Geometry: see drawing. Coordinates: mm, zero at the bounding-box minimum. Give positions to 0.01 mm unless a question says otherwise; leave off trailing zeros. Order: outer loops, then holes, each group sorted by start corner. A loop starts at its lowest first (then second) coordinate and runs counter-clockwise, first axis right, second up. Notation, with made-up numbers: M 19,0 L 67,0 A30 ccw 67,39 Z; hole C 88,65.5 d11. An arc over 180 degrees is marked long. Use a Markdown table: item, result.
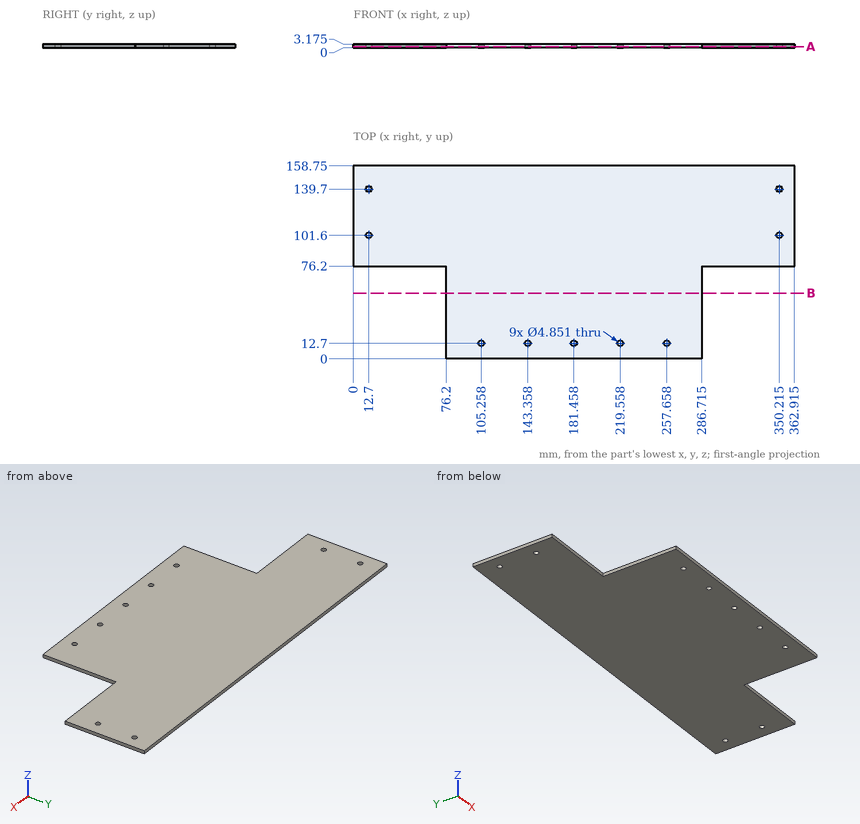
1) Cut plane B-B on y = 54. Return loops of the section in (x, z) (1 decimal).
Response values:
| item | result |
|---|---|
| outline | M 76.2,0 L 286.7,0 L 286.7,3.2 L 76.2,3.2 Z |
2) Material intervals for line 1 (X direction, y = 12.7, z = 1.5) (1 decimal); line 2 (X direction, y = 139.7, z = 2.05) (1 decimal); line 3 (X direction, y = 140.5, z = 0.5) (1 decimal), sorted ascending. Write a range as from..to.
Response values:
| item | result |
|---|---|
| line 1 | x = 76.2..102.8, 107.7..140.9, 145.8..179, 183.9..217.1, 222..255.2, 260.1..286.7 |
| line 2 | x = 0..10.3, 15.1..347.8, 352.6..362.9 |
| line 3 | x = 0..10.4, 15..347.9, 352.5..362.9 |
3) Cut plane A-A on z = 1.05. State how many separate pieces and enclosed holes the cut face has, and give its area (3 significant figures).
Response values:
| item | result |
|---|---|
| separate pieces | 1 |
| enclosed holes | 9 |
| area | 45,800 mm² |
4) First-contact query: pin 1 Ø3 at (x, y) = (350.22, 101.6) entering from -Z; pin 2 Ø1 at (y, z) = (20.5, 2) entering from +X (1 decimal). Flat tips, straight axial feed; report the tip coordinate or a pass-through.
Response values:
| item | result |
|---|---|
| pin 1 | passes through |
| pin 2 | stops at x = 286.7 |
